Can you work these out from the model? Positions are in its coordinate system, mm. Coordinates: 2 decimals unless noted, no trailing zeros. Loops run counter-clockwise (first coordinate to the right, second up) from the corner with the lowest first, then second, coordinate; pieces in that order, holes last.
```python
from build123d import *

# Parameters (mm, degrees)
F2_R = 5.08


with BuildPart() as f1:
    # F0 (on Top) → F1 (revolve)
    with BuildSketch(Plane.XY):
        Polygon((-40.960705, 10.16), (-66.756062, 37.145256), (-66.756062, 0), (78.738996, 0), (35.417151, 20.32), (24.482426, 12.7), (-30.547943, 12.7), align=None)
    revolve(axis=Axis((5.991467, 0, 0), (-1, 0, 0)))

    # F2
    f2_edges = [f1.edges().sort_by_distance(p)[0] for p in [
        (-40.960705, -10.16, 0),
        (-30.547943, -12.7, 0),
        (35.417151, -20.32, 0),
    ]]
    fillet(f2_edges, radius=F2_R)


solid = f1.part
```
(1) I'm going to push flat-ended pins straight in: pin 1 (2 mm diameter, centred on y = 16.5, z = 8.5, fed in from +X); pin 2 (5 mm diameter, centred on x = 36, y = 11, fed in from +Z); pin 3 (4 mm diameter, centred on x = -25, y = -3.5, fed in from -Z). Where does each tip first touch, or does it pass through?
Check values:
pin 1: stops at x = 41.3
pin 2: stops at z = 17.61
pin 3: stops at z = -12.61
(2) If I drill on probe 1 along Y at (x, z) = (5, -0.5); probe 2 along Y at (x, z) = (62, 3.5); probe 3 along X at (y, z) = (16.5, 14), over which ranges is the centre line in solid material (lowest first)?
Check values:
probe 1: y = -12.69 to 12.69
probe 2: y = -7.03 to 7.03
probe 3: x = -66.76 to -51.93
(3) I want a section at B-B on x = 68.5. Write out the boundary of the cut face in (y, z).
Check values:
outline: circle Ø9.61 at (0, 0)
(4) If we mould it in two halves opening along X, with no side actions, what happens to faces 1 (the conical face through (-37, 10.28, 4.26)), 2 (the conical face through (-44.474, -10.197, -9.351)), 3 (the flat face through (-66.756, -1, -1)), 4 (the conical face through (62.64, -5.993, 4.595))? For each: released by +X, released by -X, zero draft, split by the parting line, or undercut.
Check values:
face 1: undercut
face 2: undercut
face 3: released by -X
face 4: released by +X
(5) I want a section at A-A on x = 0. Write out the boundary of the cut face in (y, z), then the cut area to 3 significant figures.
Check values:
outline: circle Ø25.4 at (0, 0)
area: 507 mm2
